The drawing under review shows one solid part. Ordinate dimensions are in mm from its lowest x, y, z. A direction names the side the tool comes from. Give positions to 0.01 mm unless a question says otherwise; leave off trailing zeros. Write each loop counter-clockwise with the first axis right and the second up, starting at its lowest first coordinate (ties: lowest second). Pieces come first, ordered by that corner, then holes. Notation, with made-up numbers: M 68,3 L 77,3 A27 cw 77,23 Z; hole C 84,-38 d10. An arc over 180 degrees is marked long. Write item = value, one per line. Start each with the question number.
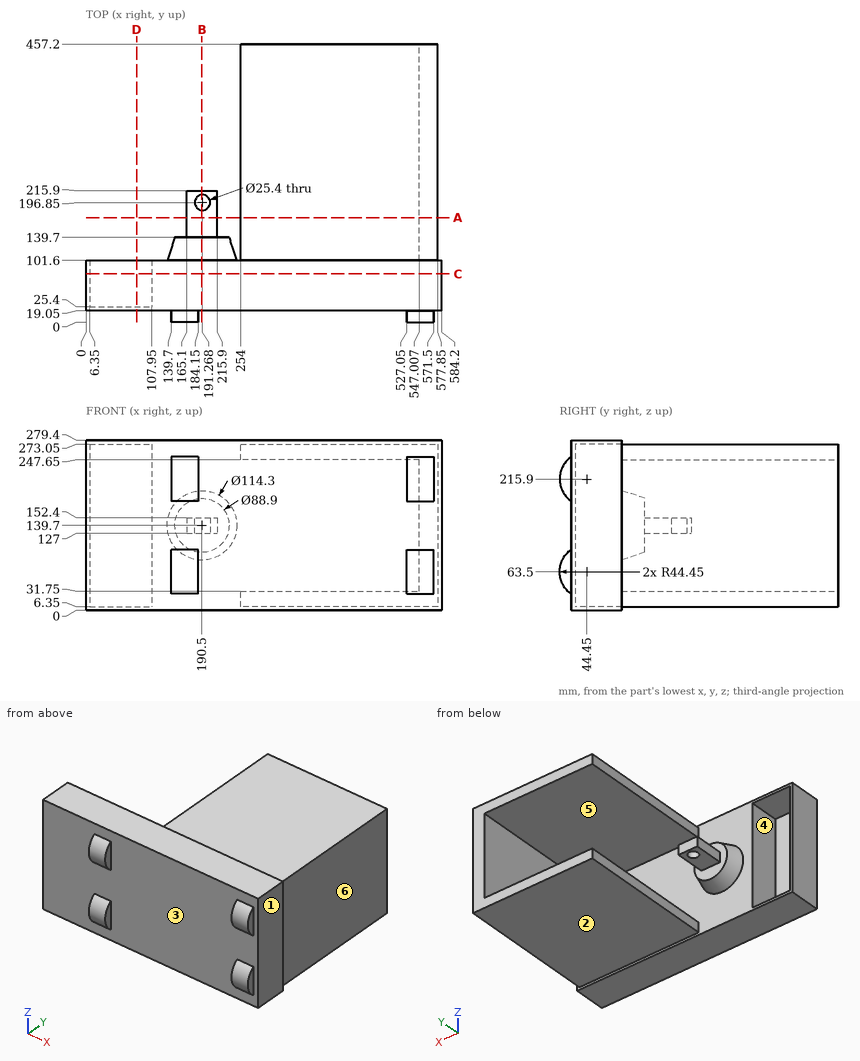
Item 1: To check wall thickness, follow probe 1 along X at (y, z) = (198, 143); probe 2 along Z at (x, y) = (538, 164.5); probe 3 along X at (y, z) = (56.5, 116.5). State the ranges of each line that lie inside material, in increasing order. Write a range as [from, to].
Item 2: We need section D-D, the plane x = 83. Write out the cut boundary in (y, z), and give its area (3 significant figures).
Item 3: We need section A-A, the plane y = 172. Write out the cut boundary in (x, z).
Item 4: The part is to be moulded in two halves that separate along X. For the marked faces 1, 2 and 3, say which applies: released by +X, released by -X, zero draft, split by the parting line, or undercut.
Item 5: For the marked faces 4, 5 and 6, list the 3-axis set-ups (+Z, -Z, +X, -X, +Y, -Y) from which the entire face can be reached by the end or side of a thin tool; tool diameter is ignored.
Item 6: Clearance check with flat-ended pins moving along their axes: P1, Ø1.5, axis at x = 303, z = 119.5, coming from the +Y side; P2, Ø9.5, axis at y = 10.5, z = 208, coming from the +X side; P3, Ø3, axis at y = 161, z = 43, coming from the +X side. State where each tip first meets the part, or that it passes through.
Item 7: We need section C-C, the plane y = 79.5. Write out the cut boundary in (x, z).
Item 8: We need section B-B, the plane x = 190.5. Write out the cut boundary in (y, z), and give its area (3 significant figures).
Worked out:
q1.probe_1 = [165.1, 178.62], [203.92, 215.9], [547.01, 577.85]
q1.probe_2 = [6.35, 31.75], [247.65, 273.05]
q1.probe_3 = [0, 6.35], [107.95, 584.2]
q2.outline = M 19.05,0 L 101.6,0 L 101.6,6.35 L 25.4,6.35 L 25.4,273.05 L 101.6,273.05 L 101.6,279.4 L 19.05,279.4 Z
q2.area = 2,740 mm²
q3.outline = M 165.1,127 L 215.9,127 L 215.9,152.4 L 165.1,152.4 Z; M 254,6.35 L 577.85,6.35 L 577.85,273.05 L 254,273.05 L 254,247.65 L 547.01,247.65 L 547.01,31.75 L 254,31.75 Z
q4.face_1 = released by +X
q4.face_2 = zero draft
q4.face_3 = undercut
q5.face_4 = +Y
q5.face_5 = -X, +Y
q5.face_6 = +Z, -Z, +X, +Y
q6.P1 = 101.6
q6.P2 = 571.5
q6.P3 = 577.85
q7.outline = M 0,0 L 584.2,0 L 584.2,279.4 L 0,279.4 Z; hole M 6.35,6.35 L 107.95,6.35 L 107.95,273.05 L 6.35,273.05 Z
q8.outline = M 19.05,0 L 101.6,0 L 101.6,82.55 L 139.7,95.25 L 139.7,127 L 184.17,127 L 184.17,152.4 L 139.7,152.4 L 139.7,184.15 L 101.6,196.85 L 101.6,279.4 L 19.05,279.4 Z; M 209.53,127 L 215.9,127 L 215.9,152.4 L 209.53,152.4 Z
q8.area = 28,200 mm²
